Part model, mm, in its own coordinate system. Give positions to 0.01 mm unless a question says otherwise; leave off trailing zeros. Write each loop counter-clockwise with the first axis right and the second up, starting at its lowest first coordinate (ties: lowest second). Pieces come first, ordered by that corner, then holes. Notation, with made-up numbers: (-9.5, 52.5) - (24.5, 52.5) arc R10 cw to (24.5, 56.5) - close; hole circle Ø6 at (26.5, 47). An arc over 180 degrees is marked (long way). Answer in a Markdown table with one row per item. Add a question column.
1. Band-saw the part on D-D on y = 0.75. State how many separate pieces and enclosed holes the cut face has, plus the area to 3 significant figures.
2. Band-saw the part on A-A on z = -50.5. Write the cut outline in (x, y), plus the area to 3 significant figures.
3. Band-saw the part on B-B on z = -7.5. Write the cut outline in (x, y), plus the area to 3 significant figures.
4. Drop a flat-ended pin along its axis: pin 1 Ø0.6 at (y, z) = (1, -27.5) entering from -X. Give the stop position or say it passes through.
5. Probe line 1 along X through (y, z) = (1.4, -2.5); line 2 along X through (y, z) = (0.55, -35.5); line 3 along X through (y, z) = (0.8, -7.5). List the from-to ranges inside material, lowest first.
6. Band-saw the part on C-C on z = -35.5. Write the cut outline in (x, y).
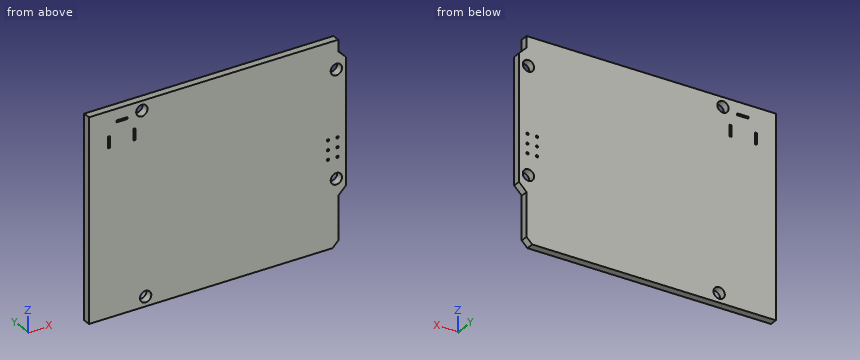
```python
from build123d import *

# Parameters (mm, degrees)
SKETCH1_R           = 1.5
BOSS_EXTRUDE1_DEPTH = 2
SKETCH5_W           = 0.5
SKETCH5_H           = 3
SKETCH5_W_2         = 3
SKETCH5_H_2         = 0.5
CUT_EXTRUDE2_DEPTH  = 3
SKETCH6_W           = 0.5
SKETCH6_H           = 0.5
CUT_EXTRUDE3_DEPTH  = 3


with BuildPart() as part:
    # Sketch1 → Boss-Extrude1 (new body)
    with BuildSketch(Plane(origin=(0, 0, 0), x_dir=(1, 0, 0), z_dir=(0, 1, 0))):
        Polygon((0, 53), (0, 0), (66, 0), (66, 3), (68, 5), (68, 38), (66, 40), (66, 51.5), (64.5, 53), align=None)
        with Locations((15, 50.5)):
            Circle(SKETCH1_R, mode=Mode.SUBTRACT)
        with Locations((14, 2.5)):
            Circle(SKETCH1_R, mode=Mode.SUBTRACT)
        with Locations((65.5, 7.5)):
            Circle(SKETCH1_R, mode=Mode.SUBTRACT)
        with Locations((65.5, 35.5)):
            Circle(SKETCH1_R, mode=Mode.SUBTRACT)
    extrude(amount=BOSS_EXTRUDE1_DEPTH)

    # Sketch5 → Cut-Extrude2 (cut, through all)
    with BuildSketch(Plane.XZ):
        with Locations((5.25, -8)):
            Rectangle(SKETCH5_W, SKETCH5_H)
        with Locations((12, -8)):
            Rectangle(SKETCH5_W, SKETCH5_H)
        with Locations((8.75, -3.25)):
            Rectangle(SKETCH5_W_2, SKETCH5_H_2)
    extrude(amount=-CUT_EXTRUDE2_DEPTH, mode=Mode.SUBTRACT)

    # Sketch6 → Cut-Extrude3 (cut, through all)
    with BuildSketch(Plane(origin=(0, 0, 0), x_dir=(-1, 0, 0), z_dir=(0, -1, 0))):
        with Locations((-63.25, 25)):
            Rectangle(SKETCH6_W, SKETCH6_H)
        with Locations((-65.75, 25)):
            Rectangle(SKETCH6_W, SKETCH6_H)
        with Locations((-65.75, 27.5)):
            Rectangle(SKETCH6_W, SKETCH6_H)
        with Locations((-65.75, 30)):
            Rectangle(SKETCH6_W, SKETCH6_H)
        with Locations((-63.25, 30)):
            Rectangle(SKETCH6_W, SKETCH6_H)
        with Locations((-63.25, 27.5)):
            Rectangle(SKETCH6_W, SKETCH6_H)
    extrude(amount=-CUT_EXTRUDE3_DEPTH, mode=Mode.SUBTRACT)


solid = part.part
```
Values:
| question | item | result |
|---|---|---|
| 1 | separate pieces | 1 |
| 1 | enclosed holes | 13 |
| 1 | area | 3,530 mm² |
| 2 | outline | (0, 0) - (13.5, 0) - (13.5, 2) - (0, 2) - close; (16.5, 0) - (66, 0) - (66, 2) - (16.5, 2) - close |
| 2 | area | 126 mm² |
| 3 | outline | (0, 0) - (5, 0) - (5, 2) - (0, 2) - close; (5.5, 0) - (11.75, 0) - (11.75, 2) - (5.5, 2) - close; (12.25, 0) - (64, 0) - (64, 2) - (12.25, 2) - close; (67, 0) - (68, 0) - (68, 2) - (67, 2) - close |
| 3 | area | 128 mm² |
| 4 | pin 1 | stops at x = 0 |
| 5 | line 1 | x = 0 to 12.5, 15.5 to 66 |
| 5 | line 2 | x = 0 to 64, 67 to 68 |
| 5 | line 3 | x = 0 to 5, 5.5 to 11.75, 12.25 to 64, 67 to 68 |
| 6 | outline | (0, 0) - (64, 0) - (64, 2) - (0, 2) - close; (67, 0) - (68, 0) - (68, 2) - (67, 2) - close |
